For this review, take the finished solid that the model builds, in its own axes (mm). Round coordinates to 2 decimals unless told otherwise and drop trailing zeros. Write each loop counter-clockwise with the first axis right and the second up, starting at its lowest first coordinate (ties: lowest second). Pieces come first, ordered by that corner, then holes. Notation, with made-up numbers: (-35, 30.5) -> (-24, 30.5) arc R18 cw to (-24, 60.5) -> close; hole circle Ø7 at (28, 58.25). An arc over 180 degrees is marked (long way). Answer as CSV lines item,"result". Start each with the question number.
Item 1: Wall thickness on probe 1 along X at (y, z) = (-15, -5); probe 2 along X at (y, z) = (8.5, 5.5); probe 3 along Z at (x, y) = (25.4, 1): over which ranges is each line inside the solid? List them lowest first. Write a range as from..to.
Item 2: Take a section at C-C on x = 152.4. Give the boundary of the cut face in (y, z).
Item 3: Take a section at D-D on x = 95. Give the boundary of the cut face in (y, z).
Item 4: For pin 1 Ø6 at (y, z) = (18.5, 17) entering from -X; pin 2 Ø3 at (y, z) = (-11, -20) entering from -X; pin 3 Ø1.5 at (x, y) = (91.5, -8.5) entering from -Z, all flat-tipped, find the tip position at first contact; note any pin that passes through.
Item 5: Take a section at B-B on y = 0. Give the boundary of the cut face in (x, z).
Item 6: Mouldability with a two-part tool opening along X and no side actions: class faces 1 (the flat face through (177.8, 0, 0)), 2 (the conical face through (0.25, -4.46, -20.08)), 3 (the cylindrical face through (146.343, -0.356, -1.907)) as +X half, -X half, draft (parallel to the pull), parting line (faces both ways), or undercut.
Item 7: Take a section at A-A on z = 0. Give the boundary of the cut face in (x, y).
```python
from build123d import *

# Parameters (mm, degrees)
F0_R     = 25.4
F1_DEPTH = 177.8
F2_SIZE  = 5.08
F4_D     = 12.7
F5_D     = 12.7


with BuildPart() as f1:
    # F0 (on Right) → F1 (new body)
    with BuildSketch(Plane.YZ):
        Circle(F0_R)
    extrude(amount=F1_DEPTH)

    # F2
    f2_edges = [f1.edges().sort_by_distance(p)[0] for p in [
        (0, -25.4, 0),
        (177.8, -25.4, 0),
    ]]
    chamfer(f2_edges, length=F2_SIZE)

    # F4 (through all)
    with Locations(Plane(origin=(0, 0, 0), x_dir=(1, 0, 0), z_dir=(0, 1, 0))):
        with Locations((152.4, 0), (25.4, 0)):
            Hole(F4_D / 2)

    # F5 (through all)
    with Locations(Plane.XZ):
        with Locations((25.4, 0), (152.4, 0)):
            Hole(F5_D / 2)


solid = f1.part
```
Output values:
1,probe 1,"x = 0..21.49, 29.31..148.49, 156.31..177.8"
1,probe 2,"x = 0..22.23, 28.57..149.23, 155.57..177.8"
1,probe 3,"z = -25.38..-6.35, 6.35..25.38"
2,outline,"(-24.59, -6.35) arc R25.4 ccw to (24.59, -6.35) -> close; (-24.59, 6.35) -> (24.59, 6.35) arc R25.4 ccw to start"
3,outline,"circle Ø50.8 at (0, 0)"
4,pin 1,"stops at x = 1.8"
4,pin 2,"stops at x = 1.01"
4,pin 3,"stops at z = -24.19"
5,outline,"(0, -20.32) -> (5.08, -25.4) -> (172.72, -25.4) -> (177.8, -20.32) -> (177.8, 20.32) -> (172.72, 25.4) -> (5.08, 25.4) -> (0, 20.32) -> close; hole circle Ø12.7 at (25.4, 0); hole circle Ø12.7 at (152.4, 0)"
6,face 1,"+X half"
6,face 2,"-X half"
6,face 3,"undercut"
7,outline,"(0, -20.32) -> (5.08, -25.4) -> (19.05, -25.4) -> (19.05, 25.4) -> (5.08, 25.4) -> (0, 20.32) -> close; (31.75, -25.4) -> (146.05, -25.4) -> (146.05, 25.4) -> (31.75, 25.4) -> close; (158.75, -25.4) -> (172.72, -25.4) -> (177.8, -20.32) -> (177.8, 20.32) -> (172.72, 25.4) -> (158.75, 25.4) -> close"
